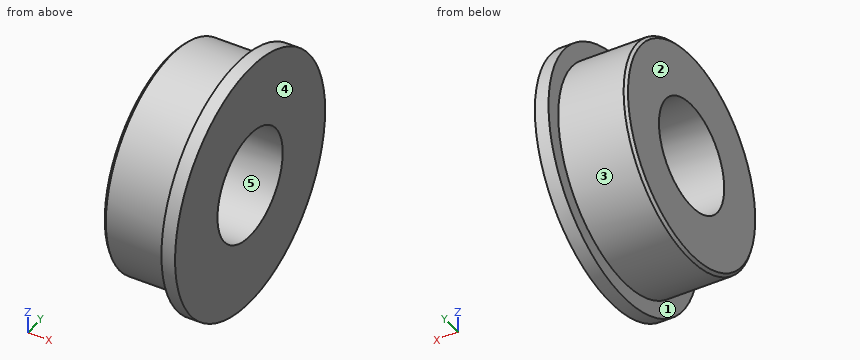
from build123d import *

# Parameters (mm, degrees)
CHAMFER_1_SIZE = 0.1


with BuildPart() as part:
    # 草图1 → 旋转1 (revolve)
    with BuildSketch(Plane.XY):
        Polygon((0, 2), (0, 4), (2.5, 4), (2.5, 4.6), (3, 4.6), (3, 2), align=None)
    revolve(axis=Axis((0, 0, 0), (1, 0, 0)))

    # 倒角1
    chamfer_1_edges = [part.edges().sort_by_distance(p)[0] for p in [
        (0, -4, 0),
    ]]
    chamfer(chamfer_1_edges, length=CHAMFER_1_SIZE)


solid = part.part
Source: CAD feature listing. Evaluate the final solid. Frame: model axes, mm. Face numbers are marked on the shaded views. A direction names the side the tool comes from. Give positions to 0.01 mm unless a question says otherwise; leave off trailing zeros. Write each loop counter-clockwise with the first axis right and the second up, starting at its lowest first coordinate (ties: lowest second). Pieces come first, ordered by that corner, then holes. Notation, with made-up numbers: M 55,6.25 L 111,6.25 A34 cw 111,44.25 Z; hole C 0,32 d6. An arc over 180 degrees is marked long. Return JSON: item names as keys, results as strings. Group by question number.
1) Cut plane C-C, the plane x = 2.15. Output: boundary loops of the cut face in (y, z), then the cut area to 3 significant figures.
2) Cut plane A-A, the plane y = 0. Output: boundary loops of the cut face in (x, z), then the cut area to 3 significant figures.
3) Draft query along Z for the marked faces 3, 4 and 5. Return one class per face: released by +Z, released by -Z, zero draft, split by the parting line, or undercut.
4) First-contact query: pin 1 Ø1.5 at (x, z) = (2.5, -2.5) entering from +Y; pin 2 Ø1 at (x, y) = (0.5, -2) entering from +Z; pin 3 Ø1 at (x, z) = (0.5, 3.5) entering from +Y. Flat tips, straight axial feed; report the tip coordinate or a pass-through.
5) Set-up query: the marked faces 1 and 2. Return all of +Z, -Z, +X, -X, +Y, -Y with unobstructed straight access to the full face (end or side cutting, diameter ignored); none if empty.
6) Ray query, L1, parallel to Z at x = 2.05, y = 0; L2, parallel to X at y = -2.5, z = -3.5; L3, parallel to Z at x = 0.45, y = -1.75. Return the intervals inside material, ascending.
Data:
{
 "1": {"outline": "C 0,0 d8; hole C 0,0 d4", "area": "37.7 mm²"},
 "2": {"outline": "M 0,-3.9 L 0.1,-4 L 2.5,-4 L 2.5,-4.6 L 3,-4.6 L 3,-2 L 0,-2 Z; M 0,2 L 3,2 L 3,4.6 L 2.5,4.6 L 2.5,4 L 0.1,4 L 0,3.9 Z", "area": "12.6 mm²"},
 "3": {"face 3": "split by the parting line", "face 4": "zero draft", "face 5": "undercut"},
 "4": {"pin 1": "stops at y = 4.25", "pin 2": "stops at z = 3.71", "pin 3": "stops at y = 2.65"},
 "5": {"face 1": "-X", "face 2": "+Z, -Z, -X, +Y, -Y"},
 "6": {"L1": "z = -4 to -2, 2 to 4", "L2": "x = 2.5 to 3", "L3": "z = -3.6 to -0.97, 0.97 to 3.6"}
}
